```python
from build123d import *

# Parameters (mm, degrees)
SKETCH1_R           = 2.54
SKETCH1_R_2         = 2.4765
BOSS_EXTRUDE1_DEPTH = 1.8796
SKETCH2_R           = 2.54
CUT_EXTRUDE1_DEPTH  = 35.760967211
CUT_EXTRUDE2_DEPTH  = 35.760967211
BOSS_EXTRUDE2_DEPTH = 6.5278
CUT_EXTRUDE4_REACH  = 37.076
SKETCH6_W           = 14.5542
SKETCH6_H           = 14.2875
SKETCH6_W_2         = 12.1666
SKETCH6_H_2         = 6.6802
BOSS_EXTRUDE3_DEPTH = 3.175
BOSS_EXTRUDE4_DEPTH = 7.2644
FILLET1_R           = 2.54
SKETCH8_W           = 9.8806
SKETCH8_H           = 10.795
CUT_EXTRUDE5_DEPTH  = 7.9375
CUT_EXTRUDE6_DEPTH  = 45.081458513


with BuildPart() as part:
    # Sketch1 → Boss-Extrude1 (new body)
    with BuildSketch(Plane.XY):
        with BuildLine():
            Line((-24.765, -24.3205), (24.765, -24.3205))
            Line((24.765, -24.3205), (24.765, 24.3205))
            Line((24.765, 24.3205), (14.605, 24.3205))
            ThreePointArc((14.605, 24.3205), (10.795, 20.5105), (6.985, 24.3205))
            Line((6.985, 24.3205), (-6.985, 24.3205))
            ThreePointArc((-6.985, 24.3205), (-10.795, 20.5105), (-14.605, 24.3205))
            Line((-14.605, 24.3205), (-24.765, 24.3205))
            Line((-24.765, 24.3205), (-24.765, -24.3205))
        make_face()
        with Locations((19.8882, 18.2245)):
            Circle(SKETCH1_R, mode=Mode.SUBTRACT)
        with Locations((16.9037, 9.652)):
            Circle(SKETCH1_R_2, mode=Mode.SUBTRACT)
        with Locations(Location((-16.9037, 9.652, 0), (0, 0, 180))):
            Circle(SKETCH1_R_2, mode=Mode.SUBTRACT)
        with Locations(Location((-19.8882, 18.2245, 0), (0, 0, 180))):
            Circle(SKETCH1_R, mode=Mode.SUBTRACT)
    extrude(amount=BOSS_EXTRUDE1_DEPTH)

    # Sketch2 → Cut-Extrude1 (cut, through all)
    with BuildSketch(Plane.XY.offset(1.8796)):
        with Locations((16.9037, -7.0231)):
            Circle(SKETCH2_R)
        with BuildLine():
            Line((16.9037, 1.532940772), (16.9037, 3.724859228))
            ThreePointArc((16.9037, 3.724859228), (16.885643629, 3.792310932), (16.866511516, 3.859465433))
            ThreePointArc((16.866511516, 3.859465433), (13.369701525, 3.722012542), (12.011049817, 6.947014704))
            ThreePointArc((12.011049817, 6.947014704), (9.433252208, -0.300277005), (16.9037, 1.532940772))
        make_face()
        with Locations((-7.9756, 1.9177)):
            Circle(SKETCH2_R)
        with Locations((-17.4752, 0.5715)):
            Circle(SKETCH2_R)
        with Locations((-6.0452, -6.9215)):
            Circle(SKETCH2_R)
        with Locations((-15.875, -6.9215)):
            Circle(SKETCH2_R)
        with Locations((7.5438, -4.8895)):
            Circle(SKETCH2_R)
    extrude(amount=-CUT_EXTRUDE1_DEPTH, mode=Mode.SUBTRACT)

    # Sketch3 → Cut-Extrude2 (cut, through all)
    with BuildSketch(Plane.XY.offset(1.8796)):
        with BuildLine():
            Line((24.765, 12.8397), (24.765, 0.6477))
            ThreePointArc((24.765, 0.6477), (22.606, 6.7437), (24.765, 12.8397))
        make_face()
    cut_extrude2 = extrude(amount=-CUT_EXTRUDE2_DEPTH, mode=Mode.SUBTRACT)

    # Mirror1: Cut-Extrude2 across plane
    add(cut_extrude2.mirror(Plane(origin=(0, 0, 0), x_dir=(0, 0, 1), z_dir=(1, 0, 0))), mode=Mode.SUBTRACT)

    # Sketch4 → Boss-Extrude2 (add, symmetric)
    with BuildSketch(Plane(origin=(0, 0, 0), x_dir=(0, 0, -1), z_dir=(1, 0, 0))):
        Polygon((-1.8796, 12.8397), (-5.0546, 11.684094506), (-5.0546, -1.4605), (-3.3528, -1.4605), (-3.3528, 10.492481318), (-1.8796, 11.028682267), align=None)
    extrude(amount=BOSS_EXTRUDE2_DEPTH, both=True)

    # Sketch5 → Cut-Extrude4 (cut, up to next)
    with BuildSketch(Plane.XY.offset(5.0546), mode=Mode.PRIVATE) as cut_extrude4_sk1:
        Polygon((-6.5278, -1.4605), (0, -1.4605), (-6.5278, 9.982294506), align=None)
    cut_extrude4_tool1 = extrude(cut_extrude4_sk1.sketch, amount=-CUT_EXTRUDE4_REACH, mode=Mode.PRIVATE) & part.part
    # Sketch5 → Cut-Extrude4 (cut, up to next)
    with BuildSketch(Plane.XY.offset(5.0546), mode=Mode.PRIVATE) as cut_extrude4_sk2:
        Polygon((6.5278, 9.982294506), (0, -1.4605), (6.5278, -1.4605), align=None)
    cut_extrude4_tool2 = extrude(cut_extrude4_sk2.sketch, amount=-CUT_EXTRUDE4_REACH, mode=Mode.PRIVATE) & part.part
    add(cut_extrude4_tool1.solids().sort_by_distance((-4.351867, 2.353765, 5.0546))[0], mode=Mode.SUBTRACT)
    add(cut_extrude4_tool2.solids().sort_by_distance((4.351867, 2.353765, 5.0546))[0], mode=Mode.SUBTRACT)

    # Sketch6 → Boss-Extrude3 (add)
    with BuildSketch(Plane.XY.offset(1.8796)):
        with Locations((0, -17.17675)):
            Rectangle(SKETCH6_W, SKETCH6_H)
        with Locations((0, -14.5669)):
            Rectangle(SKETCH6_W_2, SKETCH6_H_2, mode=Mode.SUBTRACT)
    extrude(amount=BOSS_EXTRUDE3_DEPTH)

    # Sketch7 → Boss-Extrude4 (add, symmetric)
    with BuildSketch(Plane(origin=(0, 0, 0), x_dir=(0, 0, -1), z_dir=(1, 0, 0))):
        Polygon((-5.0546, -18.7833), (-12.7, -18.7833), (-12.7, -24.3205), (-11.1125, -24.3205), (-11.1125, -27.4955), (-1.5875, -27.4955), (-1.5875, -24.3205), (-5.0546, -24.3205), align=None)
    extrude(amount=BOSS_EXTRUDE4_DEPTH, both=True)

    # Fillet1
    fillet1_edges = [part.edges().sort_by_distance(p)[0] for p in [
        (0, -18.7833, 12.7),
        (0, -27.4955, 11.1125),
    ]]
    fillet(fillet1_edges, radius=FILLET1_R)

    # Sketch8 → Cut-Extrude5 (cut)
    with BuildSketch(Plane.XZ.offset(27.4955)):
        with Locations((0, 5.3975)):
            Rectangle(SKETCH8_W, SKETCH8_H)
    extrude(amount=-CUT_EXTRUDE5_DEPTH, mode=Mode.SUBTRACT)

    # Sketch9 → Cut-Extrude6 (cut, through all)
    with BuildSketch(Plane.ZY.offset(7.2644)):
        with BuildLine():
            Line((5.207, -24.4729), (1.5875, -24.4729))
            Line((1.5875, -24.4729), (1.5875, -25.7175))
            Line((1.5875, -25.7175), (5.207, -25.7175))
            ThreePointArc((5.207, -25.7175), (5.8293, -25.0952), (5.207, -24.4729))
        make_face()
    extrude(amount=-CUT_EXTRUDE6_DEPTH, mode=Mode.SUBTRACT)


solid = part.part
```
Can you work these out from the model? Positions are in its coordinate system, mm. A direction names the side the tool comes from. Give positions to 0.01 mm unless a question says otherwise; leave off trailing zeros. Loops run counter-clockwise (first coordinate to the right, second up) from the corner with the lowest first, then second, coordinate; pieces in that order, holes last. Notation, with made-up numbers: M 36,40 L 88,40 A34 ccw 88,76 Z; hole C 20.25,46 d4. An arc over 180 degrees is marked long. One line per question, with ' | ' between items. Start each with the question number.
Q1. If I drill on line 1 (Z direction, x = 1, y = 7.5); line 2 (Y direction, x = 15.5, z = 1.75); line 3 (Z direction, x = 21, y = -23.5), over which ranges is the centre line in solid material (lowest first)? Write a range as from..to.
Q2. If we section it at C-C (z = 7.75): Please give me the cut outline in (x, y), plus the area to 3 significant figures.
Q3. If we section it at A-A (y = 17): Please give me the cut outline in (x, z) (3 decimals), plus the area to 3 significant figures.
Q4. For faces 1 (the flat face through (6, -24.473, 3)), 2 (the flat face through (-4.94, -24, 5)), 3 (the flat face through (-6, -27, 1.588)), 4 (the flat face through (0, -17.907, 3)), which set-ups out of +Z, -Z, +X, -X, +Y, -Y let a thin tool reach every point of the face, with its end or its side?
Q5. If we section it at B-B (x = -8): Please give me the cut outline in (y, z), plus the area to 3 significant figures.
Q6. If we mould it in two halves opening along Y, with no side actions, what happens to faces 5 (the cylindrical face through (0.1, -25.59, 11.03)), 6 (the flat face through (16.904, 3, 1)), 7 (the flat face through (0, -18.783, 8)), 8 (the flat face through (-7.264, -23, 8))? For each: +Y half, -Y half, draft (parallel to the pull), parting line (faces both ways), or undercut.
Q7. For pin 1 Ø3 at (x, z) = (2, 7.5) entering from -Y; pin 2 Ø5.5 at (x, y) = (1, -15.5) entering from +Z; pin 3 Ø8 at (x, y) = (-17.48, 0.57) entering from -Z; pin 4 Ø3 at (x, y) = (-16.9, 9.65) entering from -Z, each with a flat end and sliding along its axis, tell me the tip position at first contact or that it passes through.
Q8. If we section it at D-D (y = -22): Please give me the cut outline in (x, z) (3 decimals).
Computed:
1) line 1: z = 0..1.88, 3.35..5.05 | line 2: y = -24.32..-9.14, -4.91..-0.7, 3.28..7.61, 11.69..24.32 | line 3: z = 0..1.88
2) outline: M -7.26,-27.5 L -4.94,-27.5 L -4.94,-19.56 L 4.94,-19.56 L 4.94,-27.5 L 7.26,-27.5 L 7.26,-18.78 L -7.26,-18.78 Z | area: 48.2 mm²
3) outline: M -24.765,0 L -22.114,0 L -22.114,1.88 L -24.765,1.88 Z; M -17.663,0 L 17.663,0 L 17.663,1.88 L -17.663,1.88 Z; M 22.114,0 L 24.765,0 L 24.765,1.88 L 22.114,1.88 Z | area: 76.4 mm²
4) face 1: -Z, +X, -X | face 2: -Z, -Y | face 3: -Z, +X, -X, -Y | face 4: +Z
5) outline: M -24.32,0 L -8.54,0 L -8.54,1.88 L -24.32,1.88 Z; M -5.3,0 L -0.62,0 L -0.62,1.88 L -5.3,1.88 Z; M 4.46,0 L 21.73,0 L 21.73,1.88 L 4.46,1.88 Z | area: 70.9 mm²
6) face 5: -Y half | face 6: undercut | face 7: +Y half | face 8: draft
7) pin 1: stops at y = -19.56 | pin 2: stops at z = 5.05 | pin 3: stops at z = 0 | pin 4: passes through
8) outline: M -24.765,0 L -4.94,0 L -4.94,10.795 L 4.94,10.795 L 4.94,0 L 24.765,0 L 24.765,1.88 L 7.277,1.88 L 7.277,5.055 L 7.264,5.055 L 7.264,12.7 L -7.264,12.7 L -7.264,5.055 L -7.277,5.055 L -7.277,1.88 L -24.765,1.88 Z
